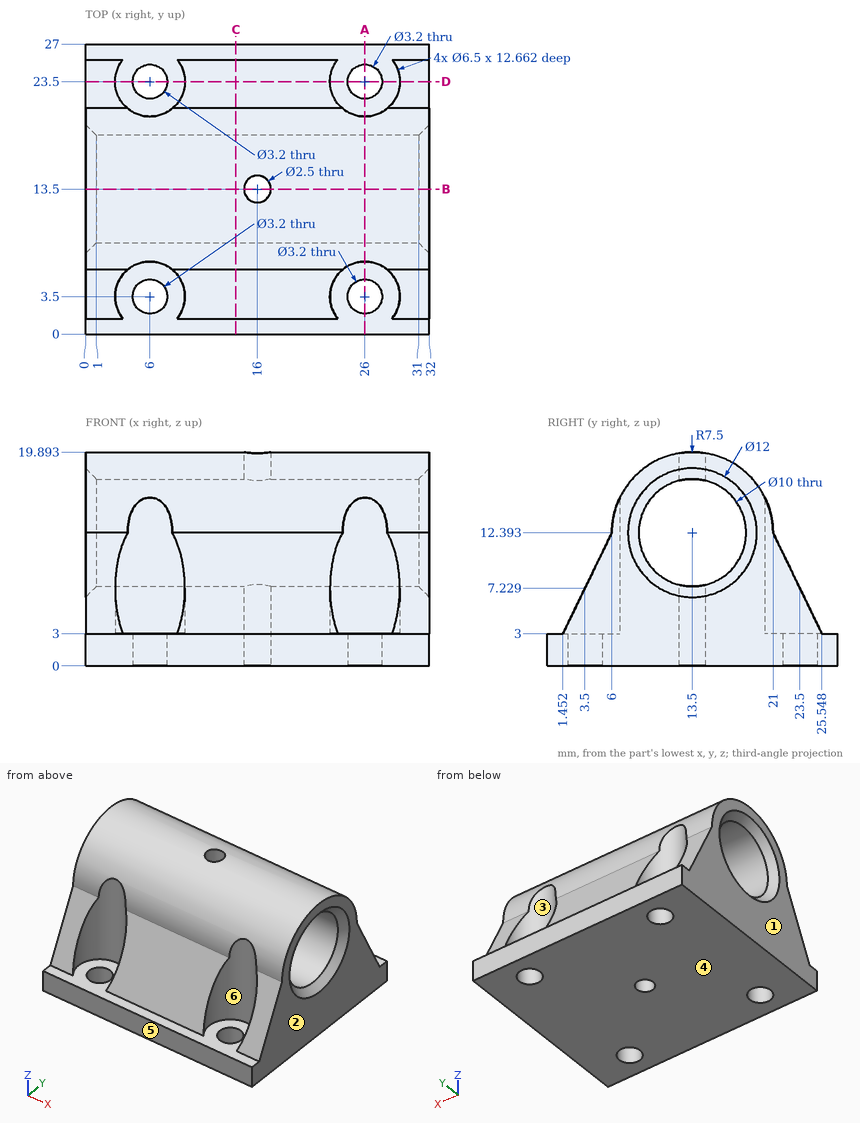
Check sheet for the drawn part. Datum: minimum x, y, z corner. Units: mm. A direction names the side the tool comes from. Give positions to 0.01 mm unless a question says otherwise; leave off trailing zeros. Order: outer loops, then holes, each group sorted by start corner. A loop starts at its lowest first (then second) coordinate and runs counter-clockwise, first axis right, second up. Notation, with made-up numbers: (85.25, -1.75) - (102.25, -1.75) arc R20 cw to (102.25, 34.25) - close; hole circle Ø8 at (-23.5, -40). An arc over 180 degrees is marked (long way). Answer in a Markdown table with one row per item. Add a question column.
Q1. Cross-section at A-A, the plane x = 26. Enter the section's corners in (y, z).
Q2. Cross-section at C-C, the plane x = 14. Enter the section's corners in (y, z).
Q3. Cross-section at D-D, the plane y = 23.5. Enter the section's corners in (x, z), then the cut area to 3 significant figures.
Q4. Mould release check, pull along X, two halves, no side actions. Record for the marked faces 1, 2, 3 and 4: pulls with the +X half, pulls with the -X half, needs draft (parallel to the pull), parting line crosses it, or undercut.
Q5. Gauge pin test, flat ends, axial feed: pin 1 (10 mm diameter, centred on x = 6.5, y = 20, fed in from +Z); pin 2 (3 mm diameter, centred on x = 6, y = 23.5, fed in from +Z); pin 3 (10.5 mm diameter, centred on x = 26, y = 3.5, fed in from +Z); pin 4 (1 mm diameter, centred on x = 16.5, z = 13.5, fed in from -Y) (1 decimal). Record the tip position at first contact, or that the pin passes through.
Q6. Material ranges on probe 1 along X at (y, z) = (3.5, 0.7); probe 2 along Y at (x, z) = (6, 1.5); probe 3 along X at (y, z) = (13.5, 19.25), recorded low to high. Write a range as from..to.
Q7. Tool access check on the marked faces 5 and 6. Record the directions out of +Z, -Z, +X, -X, +Y, -Y that give a thin tool (end or side, any length) a straight path to the whole face; none if there is none.
Q8. Cross-section at B-B, the plane y = 13.5. Enter the section's corners in (x, z).
Check values:
| question | item | result |
|---|---|---|
| 1 | outline | (0, 0) - (1.9, 0) - (1.9, 3) - (0, 3) - close; (5.1, 0) - (21.9, 0) - (21.9, 3) - (20.25, 3) - (20.25, 15.66) arc R7.5 ccw to (6.75, 15.66) - (6.75, 3) - (5.1, 3) - close; (25.1, 0) - (27, 0) - (27, 3) - (25.1, 3) - close; hole circle Ø10 at (13.5, 12.39) |
| 2 | outline | (0, 0) - (27, 0) - (27, 3) - (25.55, 3) - (21, 12.39) arc R7.5 ccw to (6, 12.39) - (1.45, 3) - (0, 3) - close; hole circle Ø10 at (13.5, 12.39) |
| 3 | outline | (0, 0) - (4.4, 0) - (4.4, 3) - (2.75, 3) - (2.75, 7.23) - (0, 7.23) - close; (7.6, 0) - (24.4, 0) - (24.4, 3) - (22.75, 3) - (22.75, 7.23) - (9.25, 7.23) - (9.25, 3) - (7.6, 3) - close; (27.6, 0) - (32, 0) - (32, 7.23) - (29.25, 7.23) - (29.25, 3) - (27.6, 3) - close |
| 3 | area | 157 mm^2 |
| 4 | face 1 | pulls with the -X half |
| 4 | face 2 | pulls with the +X half |
| 4 | face 3 | undercut |
| 4 | face 4 | needs draft |
| 5 | pin 1 | stops at z = 19.74 |
| 5 | pin 2 | passes through |
| 5 | pin 3 | stops at z = 18.2 |
| 5 | pin 4 | stops at y = 6 |
| 6 | probe 1 | x = 0..4.4, 7.6..24.4, 27.6..32 |
| 6 | probe 2 | y = 0..1.9, 5.1..21.9, 25.1..27 |
| 6 | probe 3 | x = 0..14.75, 17.25..32 |
| 7 | face 5 | +Z, -Z, +X, -X, -Y |
| 7 | face 6 | +Z |
| 8 | outline | (0, 0) - (14.75, 0) - (14.75, 7.39) - (1, 7.39) - (0, 6.39) - close; (0, 18.39) - (1, 17.39) - (14.75, 17.39) - (14.75, 19.89) - (0, 19.89) - close; (17.25, 0) - (32, 0) - (32, 6.39) - (31, 7.39) - (17.25, 7.39) - close; (17.25, 17.39) - (31, 17.39) - (32, 18.39) - (32, 19.89) - (17.25, 19.89) - close |
